Drawing for the job (mm, zero at the part's lowest x, y, z). A direction names the side the tool comes from. Coordinates: 2 decimals unless noted, no trailing zeros. Write each loop counter-clockwise with the first axis right and the second up, starting at its lowest first coordinate (ties: lowest second). Pieces come first, ordered by that corner, then holes.
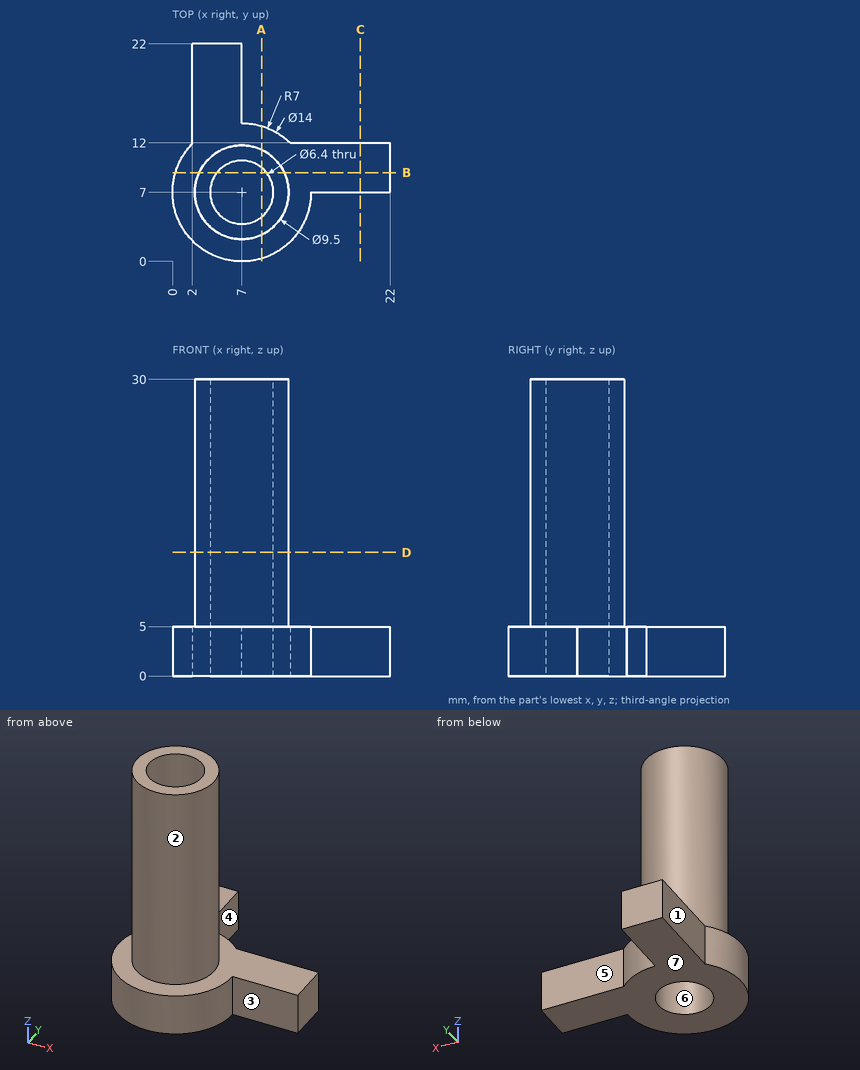
Item 1: Saw through at C-C, the plane x = 19. Write the cut outline in (y, z), and give its area (3 significant figures).
Item 2: Flat gauge pins, fed straight in: pin 1 Ø6 at (x, z) = (5, 11) entering from -Y; pin 2 Ø3 at (y, z) = (12, 3.5) entering from -X; pin 3 Ø2.5 at (x, z) = (19, 2.5) entering from -Y; pin 4 Ø5 at (x, y) = (17.5, 3) entering from -Z. Where does each tip first touch, or does it go through?
Item 3: Saw through at B-B, the plane y = 9. Write the cut outline in (x, z).
Item 4: Two-plate mould, pull along Y, no slides. Class the marked faces 5, 6 and 7: +Y half, -Y half, draft (parallel to the pull), parting line (faces both ways), or undercut.
Item 5: Wall check: line 1 along Y through (x, z) = (7, 13.25); line 2 along Y through (x, z) = (6, 12.25); line 3 along Z through (x, y) = (19, 11). Give the ranges that are in metal, low to high.
Item 6: Saw through at A-A, the plane x = 9. Write the cut outline in (y, z).
Item 7: Which spindle directions (+Z, -Z, +X, -X, +Y, -Y) get a long thin tool onto all of the face, cutting with end or side? Do the marked faces 1, 2, 3 and 4. Say none if no direction does.
Item 8: Saw through at D-D, the plane z = 12.5. Write the cut outline in (x, y).
Working result:
1. outline: (7, 0) - (12, 0) - (12, 5) - (7, 5) - close
1. area: 25.0 mm2
2. pin 1: stops at y = 2.25
2. pin 2: stops at x = 0.94
2. pin 3: stops at y = 7
2. pin 4: passes through
3. outline: (0.29, 0) - (4.5, 0) - (4.5, 30) - (2.69, 30) - (2.69, 5) - (0.29, 5) - close; (9.5, 0) - (22, 0) - (22, 5) - (11.31, 5) - (11.31, 30) - (9.5, 30) - close
4. face 5: +Y half
4. face 6: undercut
4. face 7: draft
5. line 1: y = 2.25 to 3.8, 10.2 to 11.75
5. line 2: y = 2.36 to 3.96, 10.04 to 11.64
5. line 3: z = 0 to 5
6. outline: (0.29, 0) - (4.5, 0) - (4.5, 30) - (2.69, 30) - (2.69, 5) - (0.29, 5) - close; (9.5, 0) - (13.71, 0) - (13.71, 5) - (11.31, 5) - (11.31, 30) - (9.5, 30) - close
7. face 1: +Z, -Z, -X, +Y
7. face 2: +Z
7. face 3: +Z, -Z, +X, -Y
7. face 4: +Z, -Z, +X, +Y
8. outline: circle Ø9.5 at (7, 7); hole circle Ø6.4 at (7, 7)
